from build123d import *

# Parameters (mm, degrees)
F0_R     = 5.461
F1_DEPTH = 12.7
F2_R     = 29.5275
F2_R_2   = 19.05
F3_DEPTH = 20.6248
F4_R     = 21.59
F5_DEPTH = 5.334
F6_R     = 19.05
F7_DEPTH = 25.4


with BuildPart() as f1:
    # F0 (on Top) → F1 (new body)
    with BuildSketch(Plane.XY):
        with BuildLine():
            ThreePointArc((0, 12.7), (3.719744, 3.719744), (12.7, 0))
            Line((12.7, 0), (63.5, 0))
            ThreePointArc((63.5, 0), (72.480256, 3.719744), (76.2, 12.7))
            Line((76.2, 12.7), (76.2, 63.5))
            ThreePointArc((76.2, 63.5), (72.480256, 72.480256), (63.5, 76.2))
            Line((63.5, 76.2), (12.7, 76.2))
            ThreePointArc((12.7, 76.2), (3.719744, 72.480256), (0, 63.5))
            Line((0, 63.5), (0, 12.7))
        make_face()
        with Locations((11.43, 11.43)):
            Circle(F0_R, mode=Mode.SUBTRACT)
        with Locations((64.77, 11.43)):
            Circle(F0_R, mode=Mode.SUBTRACT)
        with Locations((11.43, 64.77)):
            Circle(F0_R, mode=Mode.SUBTRACT)
        with Locations((64.77, 64.77)):
            Circle(F0_R, mode=Mode.SUBTRACT)
    extrude(amount=F1_DEPTH)

    # F2 (on face) → F3 (join)
    with BuildSketch(Plane.XY.offset(12.7)):
        with Locations((38.1, 38.1)):
            Circle(F2_R)
        with Locations((38.1, 38.1)):
            Circle(F2_R_2, mode=Mode.SUBTRACT)
    extrude(amount=F3_DEPTH)

    # F4 (on face) → F5 (cut)
    with BuildSketch(Plane.XY.offset(33.3248)):
        with Locations((38.1, 38.1)):
            Circle(F4_R)
    extrude(amount=-F5_DEPTH, mode=Mode.SUBTRACT)

    # F6 (on face) → F7 (cut)
    with BuildSketch(Plane.XY.offset(12.7)):
        with Locations((38.1, 38.1)):
            Circle(F6_R)
    extrude(amount=-F7_DEPTH, mode=Mode.SUBTRACT)


solid = f1.part
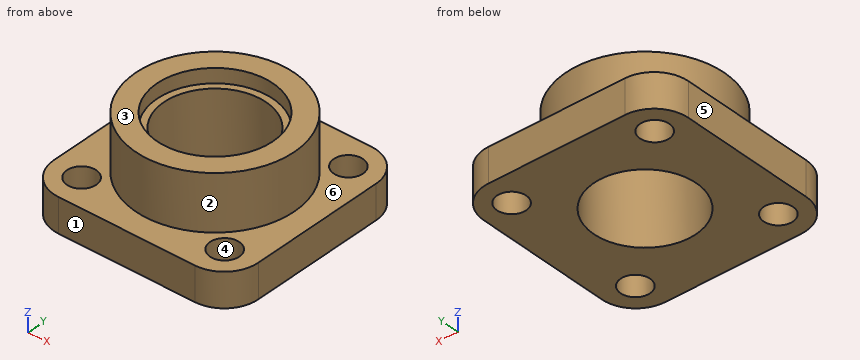
Can you work these out from the model? Positions are in its coordinate system, mm. Face numbers are marked on the shaded views. A direction names the side the tool comes from. Coordinates: 2 decimals unless noted, no trailing zeros. Loops run counter-clockwise (first coordinate to the right, second up) from the corner with the lowest first, then second, coordinate; pieces in that order, holes last. Notation, with made-up numbers: (42.5, -0.5) - (50.5, -0.5) arc R19 cw to (50.5, 18.5) - close; hole circle Ø11 at (25.5, -25.75). An arc over 180 degrees is marked (long way). Answer as a JSON object with one key per item and string values. Group by question number.
Item 1: If we section it at B-B (x = 38.1): List the corners of the cut face in (y, z) for me, plus the area to 3 significant figures.
Item 2: If we section it at A-A (z = 5): List the corners of the cut face in (x, y) for me.
Item 3: On a 3-axis mill with a long thin cutter (end or side, diameter ignored), from which of +Z, -Z, +X, -X, +Y, -Y can I reach the whole of each face in a straight line? I mean the marked faces 5 and 6. Say none if no direction works.
Item 4: For pin 1 (12 mm diameter, centred on x = 14.5, z = 26, fed in from +Y); pin 2 (3 mm diameter, centred on x = 42, z = 30, fed in from -Y); pin 3 (3 mm diameter, centred on y = 49, z = 25, fed in from -X), each with a flat end and sliding along its axis, tell me the tip position at first contact or that it passes through.
Item 5: If I drill on L1, parallel to Y at x = 38, z = 30; L2, parallel to X at y = 65.5, z = 2.5; L3, parallel to Y at x = 11, z = 10, over which ranges is the centre line in solid material (lowest first)? Write a range as from..to.
Item 6: If we mould it in two halves opening along Y, with no side actions, what happens to the marked faces 1, 2, 3 and 4? For each: released by +Y, released by -Y, zero draft, split by the parting line, or undercut.
Item 7: If we section it at D-D (x = 65): List the corners of the cut face in (y, z) for me, plus the area to 3 significant figures.
Returned:
{
 "1": {"outline": "(0, 0) - (19.05, 0) - (19.05, 27.99) - (16.51, 27.99) - (16.51, 33.32) - (8.57, 33.32) - (8.57, 12.7) - (0, 12.7) - close; (57.15, 0) - (76.2, 0) - (76.2, 12.7) - (67.63, 12.7) - (67.63, 33.32) - (59.69, 33.32) - (59.69, 27.99) - (57.15, 27.99) - close", "area": "889 mm²"},
 "2": {"outline": "(0, 12.7) arc R12.7 ccw to (12.7, 0) - (63.5, 0) arc R12.7 ccw to (76.2, 12.7) - (76.2, 63.5) arc R12.7 ccw to (63.5, 76.2) - (12.7, 76.2) arc R12.7 ccw to (0, 63.5) - close; hole circle Ø10.92 at (11.43, 11.43); hole circle Ø10.92 at (11.43, 64.77); hole circle Ø38.1 at (38.1, 38.1); hole circle Ø10.92 at (64.77, 11.43); hole circle Ø10.92 at (64.77, 64.77)"},
 "3": {"face 5": "+Z, -Z, -X, +Y, -Y", "face 6": "+Z"},
 "4": {"pin 1": "stops at y = 61.81", "pin 2": "stops at y = 8.67", "pin 3": "stops at x = 10.11"},
 "5": {"L1": "y = 8.57..16.51, 59.69..67.63", "L2": "x = 0.16..6.02, 16.84..59.36, 70.18..76.04", "L3": "y = 0.11..5.99, 16.87..59.33, 70.21..76.09"},
 "6": {"face 1": "released by -Y", "face 2": "split by the parting line", "face 3": "zero draft", "face 4": "undercut"},
 "7": {"outline": "(0.09, 0) - (5.97, 0) - (5.97, 12.7) - (0.09, 12.7) - close; (16.89, 0) - (59.31, 0) - (59.31, 12.7) - (50.28, 12.7) - (50.28, 33.32) - (25.92, 33.32) - (25.92, 12.7) - (16.89, 12.7) - close; (70.23, 0) - (76.11, 0) - (76.11, 12.7) - (70.23, 12.7) - close", "area": "1,190 mm²"}
}
